Can you work these out from the drawing? Everything is in mm from the part's minimum corner. A direction names the side the tool comes from. Round coordinates to 2 decimals unless told otherwise and drop trailing zeros. Order: outer loops, then holes, each group sorted by start corner. A loop starts at its lowest first (then second) coordinate and runs counter-clockwise, first axis right, second up. Notation, with made-up numbers: M -6,-33 L 11,-33 A11 cw 11,-21 Z; hole C -22.75,40 d7. An arc over 180 degrees is marked long. Write each question's results on one line, items separated by ' | '. Start each with the question number.
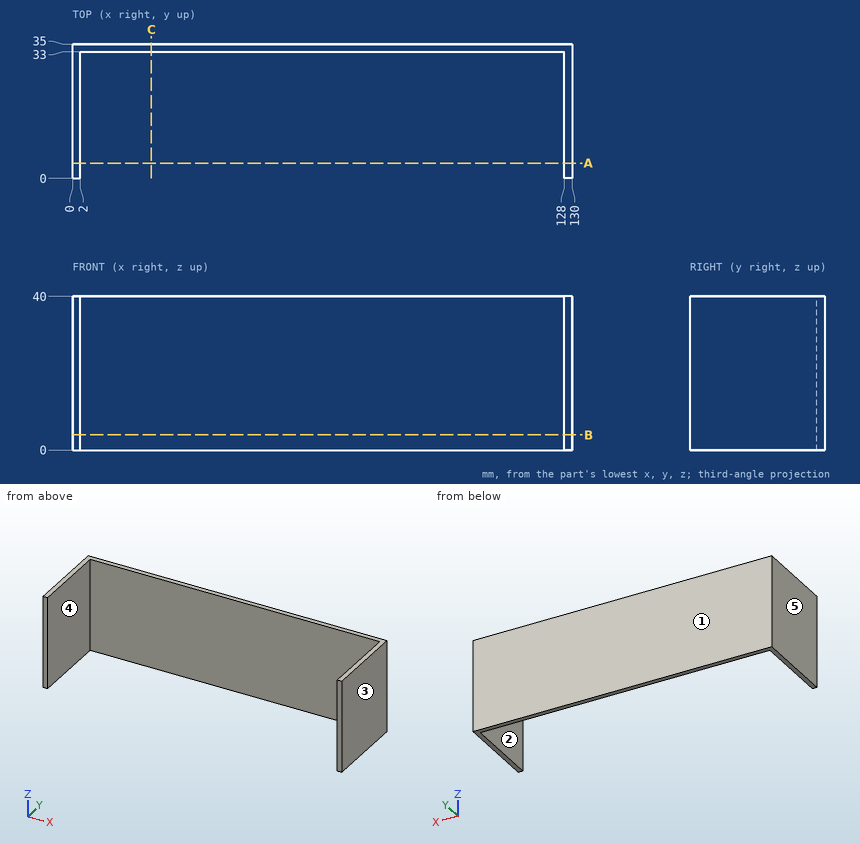
(1) I want a section at C-C on x = 20.5. Write out the boundary of the cut face in (y, z), and give its area (3 significant figures).
(2) If we mould it in two halves opening along X, with no side actions, what happens to the marked faces 1, 2 and 3? For each: pulls with the +X half, pulls with the -X half, needs draft (parallel to the pull), parting line crosses it, or undercut.
(3) On a 3-axis mill with a long thin cutter (end or side, diameter ignored), from which of +Z, -Z, +X, -X, +Y, -Y can I reach the whole of each face in a straight line? I mean the marked faces 4 and 5. Say none if no direction works.
(4) I want a section at B-B on z = 4. Write out the boundary of the cut face in (x, y), and give its area (3 significant figures).
(5) I want a section at A-A on y = 4. Write out the boundary of the cut face in (x, z).
(6) Please list where these lines run through material, in increasing order: line 1 (X direction, y = 25.5, z = 27.5); line 2 (Y direction, x = 62, z = 11).
(7) I'm going to push flat-ended pins straight in: pin 1 Ø12 at (x, z) = (49, 14.5) entering from -Y; pin 2 Ø10 at (y, z) = (18, 21.5) entering from -X. Where does each tip first touch, or does it pass through?
Solutions:
1) outline: M 33,0 L 35,0 L 35,40 L 33,40 Z | area: 80.0 mm^2
2) face 1: needs draft | face 2: undercut | face 3: pulls with the +X half
3) face 4: +Z, -Z, -Y | face 5: +Z, -Z, -X, +Y, -Y
4) outline: M 0,0 L 2,0 L 2,33 L 128,33 L 128,0 L 130,0 L 130,35 L 0,35 Z | area: 392 mm^2
5) outline: M 0,0 L 2,0 L 2,40 L 0,40 Z; M 128,0 L 130,0 L 130,40 L 128,40 Z
6) line 1: 0 to 2, 128 to 130 | line 2: 33 to 35
7) pin 1: y = 33 | pin 2: x = 0
